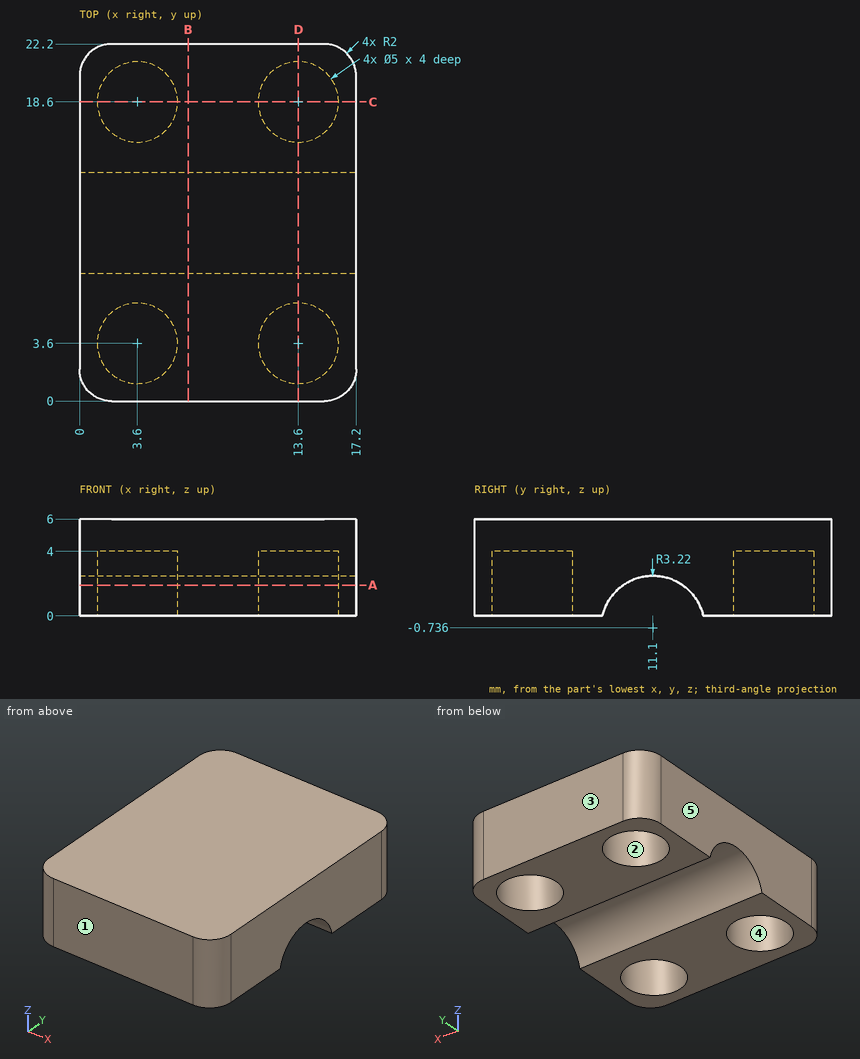
Verification items for this drawing (mm, ordinates from the low corner). A direction names the side the tool comes from. Give positions to 0.01 mm unless a question says otherwise; leave off trailing zeros. Order: outer loops, then holes, each group sorted by start corner. A loop starts at its lowest first (then second) coordinate and runs counter-clockwise, first axis right, second up.
1) Cross-section at B-B (x = 6.75). Record the boundary of the cut face in (y, z) (1 decimal).
Results are:
outline: (0, 0) - (8, 0) arc R3.2 cw to (14.2, 0) - (22.2, 0) - (22.2, 6) - (0, 6) - close
2) Draft check along X on the marked faces 3, 4 and 5. Enter one of: released by +X, released by -X, zero draft, split by the parting line, or undercut.
Results are:
face 3: zero draft
face 4: undercut
face 5: released by -X
3) Gauge pin test, flat end, axial feed: pin 1 (4 mm diameter, centred on x = 13.6, y = 3.6, fed in from -Z). Record the tip position at first contact, or that the pin passes through.
Results are:
pin 1: stops at z = 4
4) Cross-section at D-D (x = 13.6). Record the boundary of the cut face in (y, z) (1 decimal).
Results are:
outline: (0, 0) - (1.1, 0) - (1.1, 4) - (6.1, 4) - (6.1, 0) - (8, 0) arc R3.2 cw to (14.2, 0) - (16.1, 0) - (16.1, 4) - (21.1, 4) - (21.1, 0) - (22.2, 0) - (22.2, 6) - (0, 6) - close
5) Tool access check on the marked faces 1 and 2. Record the directions out of +Z, -Z, +X, -X, +Y, -Y that give a thin tool (end or side, any length) a straight path to the whole face; none if there is none.
Results are:
face 1: +Z, -Z, +X, -X, -Y
face 2: -Z
6) Material ranges on probe 1 along Y at (x, z) = (13.6, 2.75); probe 2 along Y at (x, z) = (3.6, 1.9); probe 3 along X at (y, z) = (2.25, 2.35) (1 decimal), recorded low to high.
Results are:
probe 1: y = 0 to 1.1, 6.1 to 16.1, 21.1 to 22.2
probe 2: y = 0 to 1.1, 6.1 to 9.25, 12.95 to 16.1, 21.1 to 22.2
probe 3: x = 0 to 1.5, 5.7 to 11.5, 15.7 to 17.2
7) Cross-section at C-C (y = 18.6). Record the boundary of the cut face in (x, z).
Results are:
outline: (0, 0) - (1.1, 0) - (1.1, 4) - (6.1, 4) - (6.1, 0) - (11.1, 0) - (11.1, 4) - (16.1, 4) - (16.1, 0) - (17.2, 0) - (17.2, 6) - (0, 6) - close
8) Cross-section at A-A (z = 1.9). Record the boundary of the cut face in (x, y).
Results are:
outline: (0, 2) arc R2 ccw to (2, 0) - (15.2, 0) arc R2 ccw to (17.2, 2) - (17.2, 9.25) - (0, 9.25) - close; (0, 12.95) - (17.2, 12.95) - (17.2, 20.2) arc R2 ccw to (15.2, 22.2) - (2, 22.2) arc R2 ccw to (0, 20.2) - close; hole circle Ø5 at (3.6, 3.6); hole circle Ø5 at (3.6, 18.6); hole circle Ø5 at (13.6, 3.6); hole circle Ø5 at (13.6, 18.6)
